from build123d import *

# Parameters (mm, degrees)
SKETCH1_R           = 4
SKETCH1_R_2         = 1.5
BOSS_EXTRUDE1_DEPTH = 4
BOSS_EXTRUDE2_START = 4
SKETCH1_5_R         = 4
SKETCH1_5_R_2       = 1.5
BOSS_EXTRUDE2_DEPTH = 11
SKETCH4_W           = 5.2
SKETCH4_H           = 3.2
CUT_EXTRUDE1_DEPTH  = 111.595789101


with BuildPart() as part:
    # Sketch1 → Boss-Extrude1 (new body)
    with BuildSketch(Plane(origin=(0, 0, 0), x_dir=(1, 0, 0), z_dir=(0, 1, 0))):
        with BuildLine():
            ThreePointArc((-27.172416737, 52.038463923), (-26.279661806, 51.157271509), (-25.481299644, 50.18973376))
            Line((-25.481299644, 50.18973376), (4.013837161, 10.48146126))
            ThreePointArc((4.013837161, 10.48146126), (3.535533906, 3.964466094), (-2.98146126, 3.486162839))
            Line((-2.98146126, 3.486162839), (-42.68973376, 32.981299644))
            ThreePointArc((-42.68973376, 32.981299644), (-43.657271509, 33.779661806), (-44.538463923, 34.672416737))
            Line((-44.538463923, 34.672416737), (-71.105565481, 64.486827931))
            ThreePointArc((-71.105565481, 64.486827931), (-70.710678119, 78.210678119), (-56.986827931, 78.605565481))
            Line((-56.986827931, 78.605565481), (-27.172416737, 52.038463923))
        make_face()
        with Locations((-63.639610307, 71.139610307)):
            Circle(SKETCH1_R, mode=Mode.SUBTRACT)
        with Locations((-35.355339059, 42.855339059)):
            Circle(SKETCH1_R, mode=Mode.SUBTRACT)
        with Locations((0, 7.5)):
            Circle(SKETCH1_R_2, mode=Mode.SUBTRACT)
        with Locations((-63.639610307, 71.139610307)):
            Circle(SKETCH1_R)
        with Locations((-35.355339059, 42.855339059)):
            Circle(SKETCH1_R)
        with Locations((0, 7.5)):
            Circle(SKETCH1_R_2)
    extrude(amount=BOSS_EXTRUDE1_DEPTH)

    # Sketch1_5 → Boss-Extrude2 (add)
    with BuildSketch(Plane(origin=(0, 0, 0), x_dir=(1, 0, 0), z_dir=(0, 1, 0)).offset(BOSS_EXTRUDE2_START)):
        with Locations(Location((-63.639610307, 71.139610307, 0), (0, 0, 270))):
            Circle(SKETCH1_5_R)
        with Locations(Location((-35.355339059, 42.855339059, 0), (0, 0, 270))):
            Circle(SKETCH1_5_R)
        with Locations(Location((0, 7.5, 0), (0, 0, 270))):
            Circle(SKETCH1_5_R_2)
    extrude(amount=BOSS_EXTRUDE2_DEPTH)

    # Sketch4 → Cut-Extrude1 (cut, through all)
    with BuildSketch(Plane(origin=(0, 15, 0), x_dir=(1, 0, 0), z_dir=(0, 1, 0))):
        with Locations((-35.355339059, 42.855339059)):
            Rectangle(SKETCH4_W, SKETCH4_H)
    extrude(amount=-CUT_EXTRUDE1_DEPTH, mode=Mode.SUBTRACT)


solid = part.part
The listing builds one solid part. Answer for the finished solid, in the listing's coordinates (mm). A direction names the side the tool comes from. Give positions to 0.01 mm unless a question says otherwise; leave off trailing zeros. Write each loop counter-clockwise with the first axis right and the second up, starting at its lowest first coordinate (ties: lowest second). Pieces come first, ordered by that corner, then holes. Notation, with made-up numbers: (-12.75, 23.5) - (11.25, 23.5) arc R23 cw to (11.25, 62.5) - close; hole circle Ø5 at (-36.75, 5.25). An arc over 180 degrees is marked (long way). Use a Markdown table: item, result.
1. Section D-D on z = -53 is taken. Write down the section's boundary in (x, y), plus the area to 3 significant figures.
Values follow:
| item | result |
|---|---|
| outline | (-60.87, 0) - (-28.25, 0) - (-28.25, 4) - (-60.87, 4) - close |
| area | 130 mm² |
2. Section B-B on z = -7.5 is taken. Write down the section's boundary in (x, y).
Values follow:
| item | result |
|---|---|
| outline | (-8.39, 0) - (5, 0) - (5, 4) - (1.5, 4) - (1.5, 15) - (-1.5, 15) - (-1.5, 4) - (-8.39, 4) - close |
3. A tool of negligible diameter and unlimited length cuts with its end or side. For faces 1 (the flat face through (0, 15, -8)), 2 (the flat face through (-35, 8, -41.255)), 3 (the cylindrical face through (0, 9, -9)), from which of +Z, -Z, +X, -X, +Y, -Y can it reach the whole face along a straight path? Write none if from no direction.
Values follow:
| item | result |
|---|---|
| face 1 | +Z, -Z, +X, -X, +Y |
| face 2 | +Y, -Y |
| face 3 | +Y |
4. Find the intervals of material crossed by probe 1 along Y at (x, z) = (-4, -11); probe 2 along Z at (x, y) = (-34, 13.25); probe 3 along Z at (x, y) = (-64, 11), in increasing order. Write a range as from..to.
Values follow:
| item | result |
|---|---|
| probe 1 | y = 0..4 |
| probe 2 | z = -46.62..-44.46, -41.26..-39.09 |
| probe 3 | z = -75.12..-67.16 |
5. Section A-A on y = 6.5 is taken. Write down the section's boundary in (x, z).
Values follow:
| item | result |
|---|---|
| outline | circle Ø8 at (-63.64, -71.14); circle Ø8 at (-35.36, -42.86); circle Ø3 at (0, -7.5); hole (-37.96, -44.46) - (-32.76, -44.46) - (-32.76, -41.26) - (-37.96, -41.26) - close |
6. For a pull along X with two mould halves and no side action, classify faces 4 (the flat face through (-35, 15, -41)), 5 (the cylindrical face through (-43.644, 1.972, -33.768)), 6 (the flat face through (-35, 8, -44.455)) as released by +X, released by -X, zero draft, split by the parting line, or undercut.
Values follow:
| item | result |
|---|---|
| face 4 | zero draft |
| face 5 | released by -X |
| face 6 | undercut |
7. Section C-C on x = 0 is taken. Write down the section's boundary in (y, z).
Values follow:
| item | result |
|---|---|
| outline | (0, -15.89) - (4, -15.89) - (4, -9) - (15, -9) - (15, -6) - (4, -6) - (4, -2.5) - (0, -2.5) - close |
8. Each of these flat-tipped pins is pushed along its axis until it touches: P1, Ø4, axis at x = -36, y = 6.5, coming from the -Z side; P2, Ø3, axis at y = 3.5, z = -39.5, coming from the -X side; P3, Ø6, axis at x = -20.5, z = -36.5, coming from the +Y side. Where does it stop, or does it pass through?
Values follow:
| item | result |
|---|---|
| P1 | stops at z = -46.86 |
| P2 | stops at x = -50.18 |
| P3 | stops at y = 4 |
